```python
from build123d import *

# Parameters (mm, degrees)
BOSS_EXTRUDE1_DEPTH      = 940
BOSS_EXTRUDE1_DEPTH_BACK = 940
SKETCH1_W                = 760
SKETCH1_H                = 170
FILLET1_R                = 60


with BuildPart() as part:
    # Sketch1 → Boss-Extrude1 (new, two sides: drawn at the far end of the back side and taken through both)
    with BuildSketch(Plane(origin=(0, 0, 0), x_dir=(1, 0, 0), z_dir=(0, 1, 0)).offset(-BOSS_EXTRUDE1_DEPTH_BACK)):
        Rectangle(SKETCH1_W, SKETCH1_H)
    extrude(amount=BOSS_EXTRUDE1_DEPTH + BOSS_EXTRUDE1_DEPTH_BACK)

    # Fillet1
    fillet1_edges = [part.edges().sort_by_distance(p)[0] for p in [
        (-380, 940, 0),
        (380, -940, 0),
        (0, 940, 85),
        (380, 940, 0),
        (0, 940, -85),
        (0, -940, -85),
        (-380, -940, 0),
        (-380, 0, -85),
        (380, 0, -85),
        (380, 0, 85),
        (-380, 0, 85),
        (0, -940, 85),
    ]]
    fillet(fillet1_edges, radius=FILLET1_R)


solid = part.part
```
Part model, mm, in its own coordinate system. Round coordinates to 2 decimals unless told otherwise and drop trailing zeros. Loops run counter-clockwise (first coordinate to the right, second up) from the corner with the lowest first, then second, coordinate; pieces in that order, holes last. Notation, with made-up numbers: (46, 76.5) -> (98, 76.5) arc R17 ccw to (98, 94.5) -> close; hole circle Ø11 at (-33.5, 44). An arc over 180 degrees is marked (long way). Use a Markdown table: item, result.
1) Cut at B-B, the plane z = -50.5. List the corners of the cut face in (x, y).
The answers:
| item | result |
|---|---|
| outline | (-374.31, -880) arc R54.31 ccw to (-320, -934.31) -> (320, -934.31) arc R54.31 ccw to (374.31, -880) -> (374.31, 880) arc R54.31 ccw to (320, 934.31) -> (-320, 934.31) arc R54.31 ccw to (-374.31, 880) -> close |
2) Cut at A-A, the plane y = 459. List the corners of the cut face in (x, z).
The answers:
| item | result |
|---|---|
| outline | (-380, -25) arc R60 ccw to (-320, -85) -> (320, -85) arc R60 ccw to (380, -25) -> (380, 25) arc R60 ccw to (320, 85) -> (-320, 85) arc R60 ccw to (-380, 25) -> close |
3) Drop flat-ended pins along their axis: pin 1 Ø8 at (y, z) = (-474.5, -31.5) entering from +X; pin 2 Ø1.5 at (y, z) = (65.5, 59) entering from +X; pin 3 Ø6 at (y, z) = (718.5, -38) entering from +X. Give the stop position or say it passes through.
The answers:
| item | result |
|---|---|
| pin 1 | stops at x = 379.95 |
| pin 2 | stops at x = 369.94 |
| pin 3 | stops at x = 379.16 |
4) Probe line 1 (X direction, y = 193, z = 26); line 2 (Y direction, x = 303, z = -35); line 3 (Y direction, x = -252, z = -74.5). List the from-to ranges inside material, lowest first. Write a range as [from, to].
The answers:
| item | result |
|---|---|
| line 1 | x = [-379.99, 379.99] |
| line 2 | y = [-939.16, 939.16] |
| line 3 | y = [-913.91, 913.91] |
